Could you check a few things on this model? Use its own coordinates, in mm. Face numbers are marked on the shaded views. A direction names the side the tool comes from. Coordinates: 2 decimals unless noted, no trailing zeros. Write each loop counter-clockwise with the first axis right and the second up, starting at its lowest first coordinate (ties: lowest second). Pieces come first, ordered by that corner, then holes.
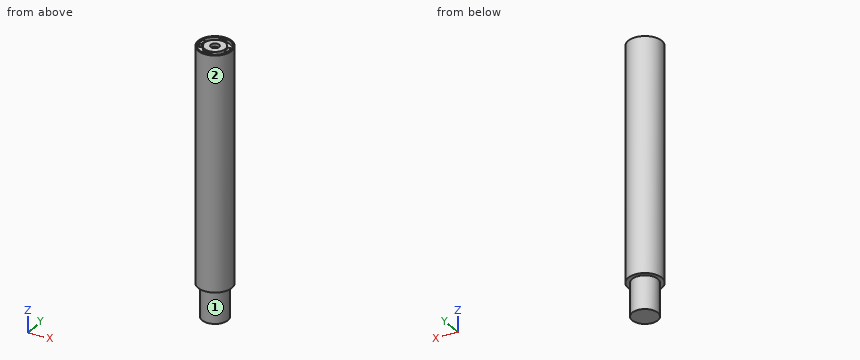
```python
from build123d import *

# Parameters (mm, degrees)
SKETCH1_R           = 2.575
BOSS_EXTRUDE1_DEPTH = 35.7
SKETCH2_R           = 2.35
CUT_EXTRUDE1_DEPTH  = 0.5
SKETCH5_R           = 1.5875
SKETCH5_R_2         = 0.635
BOSS_EXTRUDE2_DEPTH = 0.508
SKETCH6_W           = 1.016
SKETCH6_H           = 0.381
SKETCH6_W_2         = 0.381
SKETCH6_H_2         = 1.016
BOSS_EXTRUDE3_DEPTH = 0.508
SKETCH7_R           = 1.9588
BOSS_EXTRUDE4_DEPTH = 5.08


with BuildPart() as part:
    # Sketch1 → Boss-Extrude1 (new body)
    with BuildSketch(Plane.XY):
        Circle(SKETCH1_R)
    extrude(amount=-BOSS_EXTRUDE1_DEPTH)

    # Sketch2 → Cut-Extrude1 (cut)
    with BuildSketch(Plane.XY):
        Circle(SKETCH2_R)
    extrude(amount=-CUT_EXTRUDE1_DEPTH, mode=Mode.SUBTRACT)

    # Sketch5 → Boss-Extrude2 (add)
    with BuildSketch(Plane.XY):
        Circle(SKETCH5_R)
        Circle(SKETCH5_R_2, mode=Mode.SUBTRACT)
    extrude(amount=-BOSS_EXTRUDE2_DEPTH)

    # Sketch6 → Boss-Extrude3 (add)
    with BuildSketch(Plane.XY):
        with Locations((0, 1.9685)):
            Rectangle(SKETCH6_W, SKETCH6_H)
        with Locations((0, -1.9685)):
            Rectangle(SKETCH6_W, SKETCH6_H)
        with Locations((-1.9685, 0)):
            Rectangle(SKETCH6_W_2, SKETCH6_H_2)
        with Locations((1.9685, 0)):
            Rectangle(SKETCH6_W_2, SKETCH6_H_2)
    extrude(amount=-BOSS_EXTRUDE3_DEPTH)

    # Sketch7 → Boss-Extrude4 (add)
    with BuildSketch(Plane(origin=(0, 0, -35.7), x_dir=(-1, 0, 0), z_dir=(0, 0, -1))):
        Circle(SKETCH7_R)
    extrude(amount=BOSS_EXTRUDE4_DEPTH)


solid = part.part
```
1. For pin 1 (3 mm diameter, centred on x = 0.5, y = 1.5, fed in from +Z); pin 2 (1 mm diameter, centred on x = 2, y = 1.5, fed in from -Z), each with a flat end and sliding along its axis, tell me the tip position at first contact or that it passes through.
Verdict:
pin 1: stops at z = 0
pin 2: stops at z = -35.7
2. Please list where these lines run through material, in increasing order: line 1 along Z through (x, y) = (0.05, 0.5); line 2 along Z through (x, y) = (2.1, 0.25); line 3 along X through (y, z) = (-1.05, -33).
Verdict:
line 1: z = -40.78 to -0.5
line 2: z = -35.7 to 0
line 3: x = -2.35 to 2.35
3. I want a section at C-C on z = -15. Please give me the cut outline in (x, y) (3 decimals).
Verdict:
outline: circle Ø5.15 at (0, 0)
4. On a 3-axis mill with a long thin cutter (end or side, diameter ignored), from which of +Z, -Z, +X, -X, +Y, -Y can I reach the whole of each face in a straight line? I mean the marked faces 1 and 2. Say none if no direction works.
Verdict:
face 1: -Z
face 2: +Z, -Z
